Input: dimensioned drawing with shaded views. Units: mm. Origin: part minimum x, y, z. Round coordinates to 2 decimals unless told otherwise and drop trailing zeros. Write each loop counter-clockwise with the first axis right and the second up, starting at its lowest first coordinate (ties: lowest second). Pieces come first, ordered by that corner, then holes. Notation, with made-up numbers: (-19, -24) -> (9, -24) arc R31 cw to (9, 10) -> close; hole circle Ø3 at (67, -16.75). An arc over 180 degrees is marked (long way). One line per item, written item: value. Start each with the question number.
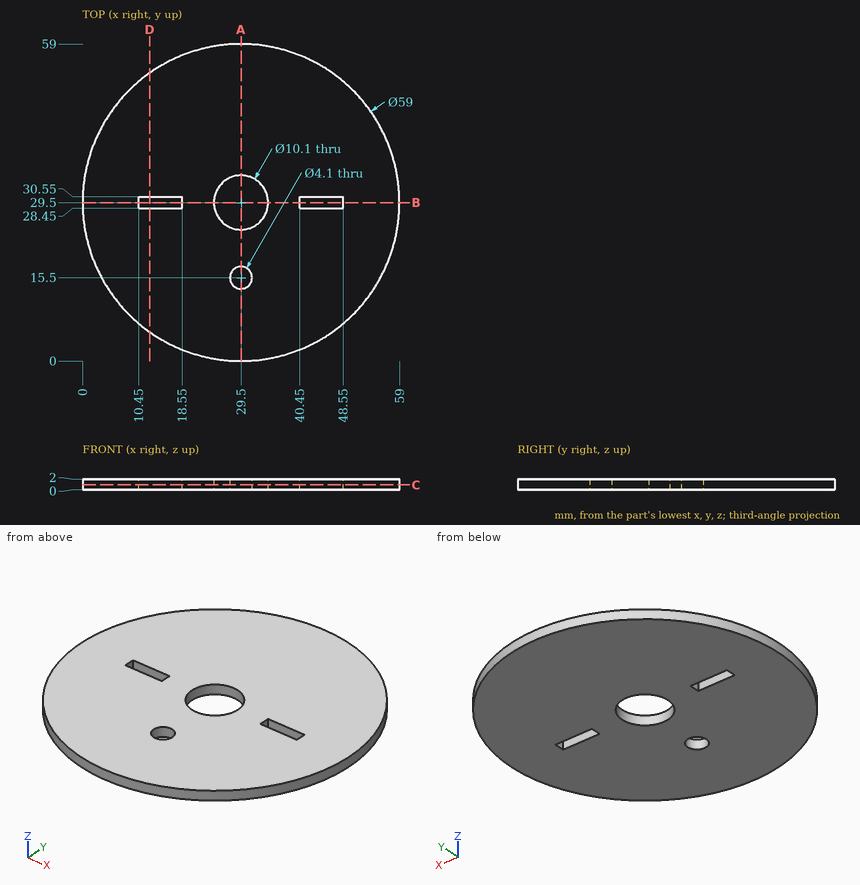
(1) Pin query (flat end, axial travel): pin 1 (1 mm diameter, centred on x = 19.5, z = 1.5, fed in from +Y); pin 2 (0.6 mm diameter, centred on y = 30, z = 1, fed in from -X); pin 3 (5 mm diameter, centred on x = 50.5, y = 25.5, fed in from -Z); pin 4 (1 mm diameter, centred on x = 42.5, z = 1, fed in from +Y). Return the tip coordinate at first contact, or that it passes through.
(2) Section query D-D (x = 12.5). Output: boundary loops of the cut face in (y, z).
(3) Section query B-B (y = 29.5). Output: boundary loops of the cut face in (x, z), and give its area (3 significant figures).
(4) Line query: probe 1 along Y at (x, z) = (29.5, 0.85); probe 2 along X at (y, z) = (30.5, 1); probe 3 along Y at (x, z) = (30.5, 1.6). Output: solid intervals per line, ascending.
(5) Section query C-C (z = 0.9). Output: boundary loops of the cut face in (x, y).
(6) Section query A-A (x = 29.5). Output: boundary loops of the cut face in (y, z), and give its area (3 significant figures).
Results list:
1. pin 1: stops at y = 57.43
1. pin 2: stops at x = 0
1. pin 3: stops at z = 0
1. pin 4: stops at y = 56.22
2. outline: (5.39, 0) -> (28.45, 0) -> (28.45, 2) -> (5.39, 2) -> close; (30.55, 0) -> (53.61, 0) -> (53.61, 2) -> (30.55, 2) -> close
3. outline: (0, 0) -> (10.45, 0) -> (10.45, 2) -> (0, 2) -> close; (18.55, 0) -> (24.45, 0) -> (24.45, 2) -> (18.55, 2) -> close; (34.55, 0) -> (40.45, 0) -> (40.45, 2) -> (34.55, 2) -> close; (48.55, 0) -> (59, 0) -> (59, 2) -> (48.55, 2) -> close
3. area: 65.4 mm^2
4. probe 1: y = 0 to 13.45, 17.55 to 24.45, 34.55 to 59
4. probe 2: x = 0.02 to 10.45, 18.55 to 24.55, 34.45 to 40.45, 48.55 to 58.98
4. probe 3: y = 0.02 to 13.71, 17.29 to 24.55, 34.45 to 58.98
5. outline: circle Ø59 at (29.5, 29.5); hole (10.45, 28.45) -> (18.55, 28.45) -> (18.55, 30.55) -> (10.45, 30.55) -> close; hole circle Ø10.1 at (29.5, 29.5); hole circle Ø4.1 at (29.5, 15.5); hole (40.45, 28.45) -> (48.55, 28.45) -> (48.55, 30.55) -> (40.45, 30.55) -> close
6. outline: (0, 0) -> (13.45, 0) -> (13.45, 2) -> (0, 2) -> close; (17.55, 0) -> (24.45, 0) -> (24.45, 2) -> (17.55, 2) -> close; (34.55, 0) -> (59, 0) -> (59, 2) -> (34.55, 2) -> close
6. area: 89.6 mm^2
